```python
from build123d import *

# Parameters (mm, degrees)
SKETCH_1_R          = 2.5
SKETCH_1_R_2        = 1.65
EXTRUDE_1_DEPTH     = 3
EXTRUDE_2_REACH     = 14.5
SKETCH_2_W          = 2
SKETCH_2_H          = 2.6
EXTRUDE_3_DEPTH     = 2
CUT_EXTRUDE_1_REACH = 4
SKETCH_4_R          = 1.65
FILLET_1_R          = 0.3
FILLET_2_R          = 0.3
FILLET_3_R          = 0.3
FILLET_4_R          = 0.3


with BuildPart() as part:
    # 草图1 → 凸台-拉伸1 (new body)
    with BuildSketch(Plane(origin=(0, 0, 0), x_dir=(1, 0, 0), z_dir=(0, 1, 0))):
        Circle(SKETCH_1_R)
        Circle(SKETCH_1_R_2, mode=Mode.SUBTRACT)
    extrude(amount=EXTRUDE_1_DEPTH)

    # 草图2 → 凸台-拉伸2 (add, up to next)
    with BuildSketch(Plane.XY.offset(10), mode=Mode.PRIVATE) as extrude_2_sk1:
        with Locations((-1.5, 1.5)):
            Rectangle(SKETCH_2_W, SKETCH_2_H)
    extrude_2_tool1 = extrude(extrude_2_sk1.sketch, amount=-EXTRUDE_2_REACH, mode=Mode.PRIVATE) - part.part
    add(extrude_2_tool1.solids().sort_by_distance((-1.5, 1.5, 10))[0])

    # 草图3 → 凸台-拉伸3 (add)
    with BuildSketch(Plane.ZY.offset(2.5)):
        with BuildLine():
            Line((10, 2.8), (10, 0.2))
            Line((10, 0.2), (10.764273601, -0.85161108))
            ThreePointArc((10.764273601, -0.85161108), (18, 1.5), (10.764273601, 3.85161108))
            Line((10.764273601, 3.85161108), (10, 2.8))
        make_face()
    extrude(amount=-EXTRUDE_3_DEPTH)

    # 草图4 → 切除-拉伸1 (cut, up to next)
    with BuildSketch(Plane(origin=(-0.5, 0, 0), x_dir=(0, 0, -1), z_dir=(1, 0, 0)), mode=Mode.PRIVATE) as cut_extrude_1_sk1:
        with Locations((-14, 1.5)):
            Circle(SKETCH_4_R)
    cut_extrude_1_tool1 = extrude(cut_extrude_1_sk1.sketch, amount=-CUT_EXTRUDE_1_REACH, mode=Mode.PRIVATE) & part.part
    add(cut_extrude_1_tool1.solids().sort_by_distance((-0.5, 1.5, 14))[0], mode=Mode.SUBTRACT)

    # 圆角1
    fillet_1_edges = [part.edges().sort_by_distance(p)[0] for p in [
        (-0.5, 1.5, 15.65),
    ]]
    fillet(fillet_1_edges, radius=FILLET_1_R)

    # 圆角2
    fillet_2_edges = [part.edges().sort_by_distance(p)[0] for p in [
        (-1.65, 3, 0),
    ]]
    fillet(fillet_2_edges, radius=FILLET_2_R)

    # 圆角3
    fillet_3_edges = [part.edges().sort_by_distance(p)[0] for p in [
        (-1.65, 0, 0),
    ]]
    fillet(fillet_3_edges, radius=FILLET_3_R)

    # 圆角4
    fillet_4_edges = [part.edges().sort_by_distance(p)[0] for p in [
        (-2.5, 1.5, 15.65),
    ]]
    fillet(fillet_4_edges, radius=FILLET_4_R)


solid = part.part
```
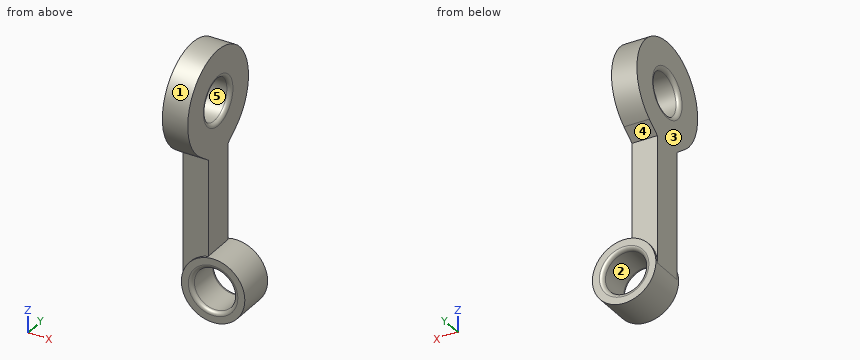
Work out the finished part from the listing and answer in its coordinate system (mm). Face numbers are marked on the shaded views. A direction names the side the tool comes from. Give positions to 0.01 mm unless a question says otherwise; leave off trailing zeros. Order: outer loops, then holes, each group sorted by start corner. A loop starts at its lowest first (then second) coordinate and runs counter-clockwise, first axis right, second up. Notation, with made-up numbers: (77.5, 8.25) - (123.5, 8.25) arc R22 ccw to (123.5, 40.25) - close; hole circle Ø4 at (56.25, 46.5). An arc over 180 degrees is marked (long way). One line per item, written item: value. Start each with the question number.
1. Which of the six approach directions +Z, -Z, +X, -X, +Y, -Y give full straight-line access (tool end or side, diameter ignored) to the marked faces 4 and 5?
2. Section B-B, the plane x = 0 is taken. Write down the section's boundary in (y, z), then the cut area to 3 significant figures.
3. Each of these flat-tipped pins is pushed along its axis until it touches: pin 1 Ø1.6 at (x, z) = (-1, 3) entering from +Y; pin 2 Ø1.6 at (x, z) = (-1.5, 5.5) entering from -Y; pin 3 Ø1 at (x, z) = (0.5, 5) entering from -Y. Where does it stop, or does it pass through?
4. Section A-A, the plane y = 1.5 is taken. Write down the section's boundary in (x, z).
5. Consider line 1 (Z direction, x = 0, y = 1.4); line 2 (X direction, y = 2.75, z = 4). Determine where each line is inside the solid, lowest interval first.
6. For a pull along Z with two mould halves and no side action, classify the marked faces 1, 2 and 3 as released by +Z, released by -Z, zero draft, split by the parting line, or undercut.
7. Section D-D, the plane z = 3.25 is taken. Write down the section's boundary in (x, y).
8. Section C-C, the plane z = 14 is taken. Write down the section's boundary in (x, y), then the cut area to 3 significant figures.
Filled sheet:
1. face 4: +X, -X, +Y
1. face 5: +X, -X
2. outline: (0, -2.5) - (3, -2.5) - (3, -1.95) arc R0.3 ccw to (2.7, -1.65) - (0.3, -1.65) arc R0.3 ccw to (0, -1.95) - close; (0, 1.95) arc R0.3 ccw to (0.3, 1.65) - (2.7, 1.65) arc R0.3 ccw to (3, 1.95) - (3, 2.5) - (0, 2.5) - close
2. area: 5.02 mm²
3. pin 1: y = 3
3. pin 2: y = 0.2
3. pin 3: through
4. outline: (-2.5, 0) arc R2.5 ccw (long way) to (-0.5, 2.45) - (-0.5, 12.05) arc R0.3 ccw to (-0.8, 12.35) - (-2.2, 12.35) arc R0.3 ccw to (-2.5, 12.05) - close; (-2.5, 15.95) arc R0.3 ccw to (-2.2, 15.65) - (-0.8, 15.65) arc R0.3 ccw to (-0.5, 15.95) - (-0.5, 18) - (-2.5, 18) - close; hole circle Ø3.3 at (0, 0)
5. line 1: -2.5 to -1.65, 1.65 to 2.5
5. line 2: -2.5 to -0.5
6. face 1: split by the parting line
6. face 2: undercut
6. face 3: zero draft
7. outline: (-2.5, 0.2) - (-0.5, 0.2) - (-0.5, 2.8) - (-2.5, 2.8) - close
8. outline: (-2.5, -2.5) - (-0.5, -2.5) - (-0.5, -0.45) arc R0.3 ccw to (-0.8, -0.15) - (-2.2, -0.15) arc R0.3 ccw to (-2.5, -0.45) - close; (-2.5, 3.45) arc R0.3 ccw to (-2.2, 3.15) - (-0.8, 3.15) arc R0.3 ccw to (-0.5, 3.45) - (-0.5, 5.5) - (-2.5, 5.5) - close
8. area: 9.32 mm²
